from build123d import *

# Parameters (mm, degrees)
F1_DEPTH = 101.6
F2_W     = 25.4
F2_H     = 12.7
F3_DEPTH = 1.27
F4_W     = 76.3398231938
F4_H     = 12.2339436784
F4_H_2   = 12.9679823294
F4_H_3   = 10.0934545674
F4_H_4   = 11.5307184484
F5_DEPTH = 16.51
F6_W     = 76.3398231938
F6_H     = 45.6335150034
F7_DEPTH = 12.7
F8_W     = 76.3398231938
F8_H     = 33.1548914642
F9_DEPTH = 10.16


with BuildPart() as f1:
    # F0 (on Right) → F1 (new body)
    with BuildSketch(Plane.YZ):
        Polygon((27.8234868258, 43.0451085358), (-48.3765131742, -33.1548914642), (27.8234868258, -33.1548914642), align=None)
    extrude(amount=F1_DEPTH)

    # F2 (on face) → F3 (cut)
    with BuildSketch(Plane(origin=(0, -7.610810855, 7.610810855), x_dir=(1, 0, 0), z_dir=(0, -0.7071067812, 0.7071067812))):
        with Locations((22.7085306913, -6.35)):
            Rectangle(F2_W, F2_H)
        with Locations((79.47403301, -6.35)):
            Rectangle(F2_W, F2_H)
    extrude(amount=-F3_DEPTH, mode=Mode.SUBTRACT)

    # F4 (on face) → F5 (cut)
    with BuildSketch(Plane(origin=(0, 27.8234868258, 0), x_dir=(-1, 0, 0), z_dir=(0, 1, 0))):
        with Locations((-51.3592674397, 19.0849541686)):
            Rectangle(F4_W, F4_H)
        with Locations((-51.3592674397, 6.4839911647)):
            Rectangle(F4_W, F4_H_2)
        with Locations((-51.3592674397, -5.0467272837)):
            Rectangle(F4_W, F4_H_3)
        with Locations((-51.3592674397, -15.8588137916)):
            Rectangle(F4_W, F4_H_4)
        with Locations((-51.3592674397, -27.38953224)):
            Rectangle(F4_W, F4_H_4)
    extrude(amount=-F5_DEPTH, mode=Mode.SUBTRACT)

    # F6 (on face) → F7 (cut)
    with BuildSketch(Plane(origin=(0, 11.3134868258, 0), x_dir=(-1, 0, 0), z_dir=(0, 1, 0))):
        with Locations((-51.3592674397, -10.3381339625)):
            Rectangle(F6_W, F6_H)
    extrude(amount=-F7_DEPTH, mode=Mode.SUBTRACT)

    # F8 (on face) → F9 (cut)
    with BuildSketch(Plane(origin=(0, -1.3865131742, 0), x_dir=(-1, 0, 0), z_dir=(0, 1, 0))):
        with Locations((-51.3592674397, -16.5774457321)):
            Rectangle(F8_W, F8_H)
    extrude(amount=-F9_DEPTH, mode=Mode.SUBTRACT)


solid = f1.part
Model file for the job. Use its own axes, mm. A direction names the side the tool comes from. Give positions to 0.01 mm unless a question says otherwise; leave off trailing zeros. Loops run counter-clockwise (first coordinate to the right, second up) from the corner with the lowest first, then second, coordinate; pieces in that order, holes last.
1) Tool access for faces 5 (the flat face through (52, -1.387, 6)), 6 (the flat face through (50, -28, -33.155)): list every direction of +Z, -Z, +X, -X, +Y, -Y with a clear straight run to the whole face (end or side of a thin tool).
2) Wall check: line 1 (X direction, y = 21, z = -14); line 2 (Z direction, x = 28.5, y = 10); line 3 (Y direction, x = 24, z = -5). Give the ranges that are in metal, low to high.
3) Pull direction X, two halves, no side cores. Call faces 1 (the flat face through (0, 6, -11)), 2 (the flat face through (10.009, -12, 3)), 3 (the flat face through (13.189, 13, -11)), 4 (the flat face through (50.09, -9.74, 5.48)): +X half, -X half, draft (parallel to the pull), parting line (faces both ways), or undercut.
4) Saw through at D-D (z = -16.5). Write the cut outline in (x, y).
5) Flat gauge pins, fed straight in: pin 1 Ø11 at (y, z) = (-13.5, 2) entering from -X; pin 2 Ø12 at (x, y) = (24.5, -17) entering from +Z; pin 3 Ø6 at (x, z) = (42.5, 8.5) entering from +Y; pin 4 Ø14 at (x, z) = (35, 18) entering from +Y. Where does each tip first touch, or does it go through?
6) Saw through at B-B (z = 3.5). Write the cut outline in (x, y).
7) Saw through at A-A (x = 55.5). Write the cut outline in (y, z).
8) Saw through at C-C (y = 20). Write the cut outline in (x, z).
Answer block:
1. face 5: -Z, +Y
1. face 6: -Z, +X, -X, +Y, -Y
2. line 1: x = 0 to 13.19, 89.53 to 101.6
2. line 2: z = 12.48 to 25.22
2. line 3: y = -20.22 to -11.55
3. face 1: -X half
3. face 2: undercut
3. face 3: undercut
3. face 4: draft
4. outline: (0, -31.72) - (101.6, -31.72) - (101.6, 27.82) - (89.53, 27.82) - (89.53, -11.55) - (13.19, -11.55) - (13.19, 27.82) - (0, 27.82) - close
5. pin 1: stops at x = 0
5. pin 2: stops at z = 2.43
5. pin 3: stops at y = -1.39
5. pin 4: stops at y = 11.31
6. outline: (0, -11.72) - (10.01, -11.72) - (10.01, -9.93) - (35.41, -9.93) - (35.41, -11.72) - (66.77, -11.72) - (66.77, -9.93) - (92.17, -9.93) - (92.17, -11.72) - (101.6, -11.72) - (101.6, 27.82) - (89.53, 27.82) - (89.53, -1.39) - (13.19, -1.39) - (13.19, 27.82) - (0, 27.82) - close
7. outline: (-48.38, -33.15) - (-11.55, -33.15) - (-11.55, 0) - (-1.39, 0) - (-1.39, 12.48) - (11.31, 12.48) - (11.31, 25.2) - (27.82, 25.2) - (27.82, 43.05) - close
8. outline: (0, -33.15) - (13.19, -33.15) - (13.19, 25.2) - (89.53, 25.2) - (89.53, -33.15) - (101.6, -33.15) - (101.6, 35.22) - (0, 35.22) - close
